from build123d import *

# Parameters (mm, degrees)
SKETCH1_R                         = 63.5
SKETCH1_R_2                       = 9.525
BOSS_EXTRUDE1_DEPTH               = 9.525
SKETCH4_R                         = 2.413
CUT_EXTRUDE1_DEPTH                = 10.525
CIRPATTERN1_COUNT                 = 8
SKETCH7_R                         = 33.02
BOSS_EXTRUDE4_DEPTH               = 4.826
SKETCH9_R                         = 33.02
CUT_EXTRUDE2_DEPTH                = 3.048
PIPE_TAP_DRILL_FOR_3_4_TAP4_D     = 23.0124
PIPE_TAP_DRILL_FOR_3_4_TAP4_DEPTH = 3.81
PIPE_TAP_DRILL_FOR_3_4_TAP4_TIP   = 6.913622455


with BuildPart() as part:
    # Sketch1 → Boss-Extrude1 (new body)
    with BuildSketch(Plane.XY):
        Circle(SKETCH1_R)
        Circle(SKETCH1_R_2, mode=Mode.SUBTRACT)
    extrude(amount=BOSS_EXTRUDE1_DEPTH)

    # Sketch4 → Cut-Extrude1 (cut, through all)
    with BuildSketch(Plane.XY.offset(9.525)):
        with Locations((49.866397767, 20.655338262)):
            Circle(SKETCH4_R)
    cut_extrude1 = extrude(amount=-CUT_EXTRUDE1_DEPTH, mode=Mode.SUBTRACT)

    # CirPattern1: Cut-Extrude1 ×8 about axis
    cirpattern1_axis = Axis((0, 0, 0), (0, 0, 1))
    for i in range(1, CIRPATTERN1_COUNT):
        add(cut_extrude1.rotate(cirpattern1_axis, i * 360 / CIRPATTERN1_COUNT), mode=Mode.SUBTRACT)

    # Sketch7 → Boss-Extrude4 (add)
    with BuildSketch(Plane.XY):
        with BuildLine():
            ThreePointArc((44.898742199, 0), (44.018213285, 2.330669915), (41.72653773, 3.308205888))
            Line((41.72653773, 3.308205888), (38.377645632, 3.308205888))
            ThreePointArc((38.377645632, 3.308205888), (36.132581602, 2.378269918), (35.202645632, 0.133205888))
            ThreePointArc((35.202645632, 0.133205888), (34.829644744, -0.48063442), (34.295865632, 0))
            add(Edge.make_bspline(
                [(34.295865632, 0), (34.29882834, 0.071916436), (34.304754577, 0.21576926), (34.311966888, 0.431642324), (34.317934755, 0.647612083), (34.327139988, 1.079917114), (34.332942166, 2.090306576), (34.279898225, 3.607362054), (34.120445155, 5.41030125), (33.960201682, 6.560746683), (33.865422793, 7.135076209), (33.865142183, 7.136775827)],
                knots=[0, 0, 0, 0, 0.000870248, 0.001740737, 0.002611466, 0.003482435, 0.006968712, 0.014826916, 0.02182843, 0.028845498, 0.028866325, 0.028866325, 0.028866325, 0.028866325], degree=3))
            add(Edge.make_bspline(
                [(33.865142183, 7.136775827), (33.7706713, 7.708973751), (33.552478291, 8.851599937), (33.138997804, 10.54970943), (32.639140351, 12.230302519), (32.054174895, 13.887355713), (31.385187056, 15.516557503), (30.633483645, 17.113645751), (29.800589951, 18.674419055), (28.8882464, 20.194747988), (27.898404875, 21.670586138), (26.833224521, 23.097980967), (25.695067067, 24.473084443), (24.486491635, 25.79216345), (23.210249051, 27.051609932), (21.869275652, 28.247950753), (20.466686605, 29.377857252), (19.005768742, 30.438154464), (17.489972932, 31.425829986), (15.922906004, 32.338042467), (14.30832223, 33.172129685), (12.650114403, 33.925616212), (10.95230451, 34.596220626), (9.219034045, 35.18186226), (7.454553956, 35.680667464), (5.663214286, 36.090975363), (3.849453494, 36.411343101), (2.017787512, 36.640550541), (0.172798549, 36.777604421), (-1.680876324, 36.82174194), (-3.538556782, 36.772433779), (-5.395531021, 36.629386524), (-7.247067665, 36.392544506), (-9.088427776, 36.062091031), (-10.914876942, 35.638449008), (-12.721697408, 35.122280961), (-14.504200214, 34.514488429), (-16.257737325, 33.816210747), (-17.977713699, 33.028823219), (-19.659599284, 32.153934663), (-21.298940898, 31.193384362), (-22.891373965, 30.149238397), (-24.43263408, 29.02378539), (-25.918568367, 27.819531655), (-27.345146601, 26.539195761), (-28.708472073, 25.185702541), (-30.004792148, 23.762176529), (-31.230508517, 22.271934869), (-32.382187085, 20.718479685), (-33.456567491, 19.105489956), (-34.450572223, 17.436812889), (-35.361315302, 15.716454831), (-36.186110516, 13.948571725), (-36.92247918, 12.137459144), (-37.568157395, 10.287541924), (-38.121102788, 8.403363415), (-38.579500717, 6.489574383), (-38.941769921, 4.550921586), (-39.206567586, 2.592236057), (-39.372793836, 0.618421113), (-39.439595611, -1.36555987), (-39.406369933, -3.354695889), (-39.272766542, -5.343940927), (-39.038689903, -7.328226707), (-38.704300556, -9.302475561), (-38.270015827, -11.261613379), (-37.736509879, -13.200582609), (-37.104713104, -15.11435526), (-36.375810853, -16.997945903), (-35.551241515, -18.846424601), (-34.632693929, -20.654929769), (-33.622104149, -22.418680905), (-32.521651558, -24.132991168), (-31.333754343, -25.793279776), (-30.061064337, -27.395084183), (-28.706461239, -28.934071999), (-27.273046228, -30.406052641), (-25.764134977, -31.806988658), (-24.18325009, -33.133006716), (-22.534112978, -34.380408214), (-20.820635184, -35.545679488), (-19.046909189, -36.625501594), (-17.217198713, -37.616759627), (-15.335928538, -38.516551562), (-13.407673866, -39.322196576), (-11.437149261, -40.031242854), (-9.429197172, -40.641474829), (-7.388776087, -41.15091985), (-5.32094834, -41.557854256), (-3.230867597, -41.86080884), (-1.123766056, -42.058573678), (0.995058608, -42.150202316), (3.120256518, -42.135015304), (5.246439066, -42.01260305), (7.368192535, -41.782828005), (9.480091844, -41.445826152), (11.576714375, -41.002007803), (13.652653862, -40.452057696), (15.702534288, -39.796934391), (17.72102376, -39.037868953), (19.702848338, -38.176362944), (21.642805765, -37.214185701), (23.535779073, -36.153370925), (25.376750026, -34.996212572), (27.16081237, -33.745260064), (28.883184839, -32.403312824), (30.539223912, -30.973414146), (32.12443625, -29.458844418), (33.634490817, -27.863113704), (35.065230621, -26.189953715), (36.412684063, -24.44330917), (37.673075861, -22.62732858), (38.842837509, -20.746354475), (39.91861725, -18.804913085), (40.897289536, -16.807703518), (41.775963949, -14.759586443), (42.55199355, -12.665572318), (43.22298264, -10.530809183), (43.786793912, -8.360570051), (44.241554967, -6.16023993), (44.571284542, -4.028278167), (44.740560267, -2.440845712), (44.813728039, -1.50376068), (44.839477521, -1.128293226), (44.857032226, -0.846470241), (44.872782179, -0.564469795), (44.886887576, -0.282309503), (44.894790326, -0.094111086), (44.898742199, 0)],
                knots=[0.028866325, 0.028866325, 0.028866325, 0.028866325, 0.035878186, 0.042926556, 0.049990663, 0.057070561, 0.064166299, 0.071277925, 0.078405484, 0.085549018, 0.092708569, 0.099884178, 0.107075882, 0.11428372, 0.121507729, 0.128747942, 0.136004396, 0.143277124, 0.150566158, 0.157871532, 0.165193276, 0.172531421, 0.179885999, 0.187257038, 0.194644569, 0.202048619, 0.209469218, 0.216906393, 0.224360171, 0.23183058, 0.239317647, 0.246821397, 0.254341857, 0.261879053, 0.269433009, 0.277003751, 0.284591303, 0.292195691, 0.299816937, 0.307455067, 0.315110103, 0.32278207, 0.33047099, 0.338176886, 0.345899781, 0.353639698, 0.361396658, 0.369170685, 0.376961799, 0.384770023, 0.392595378, 0.400437886, 0.408297568, 0.416174444, 0.424068536, 0.431979864, 0.439908449, 0.447854312, 0.455817472, 0.463797949, 0.471795764, 0.479810937, 0.487843486, 0.495893432, 0.503960795, 0.512045592, 0.520147845, 0.52826757, 0.536404789, 0.544559519, 0.552731779, 0.560921587, 0.569128963, 0.577353925, 0.58559649, 0.593856678, 0.602134505, 0.610429991, 0.618743153, 0.627074009, 0.635422576, 0.643788872, 0.652172916, 0.660574723, 0.668994312, 0.677431699, 0.685886903, 0.69435994, 0.702850826, 0.71135958, 0.719886217, 0.728430756, 0.736993211, 0.745573601, 0.754171941, 0.762788249, 0.771422539, 0.78007483, 0.788745137, 0.797433476, 0.806139864, 0.814864316, 0.823606849, 0.832367479, 0.841146221, 0.849943091, 0.858758106, 0.86759128, 0.87644263, 0.885312171, 0.894199918, 0.903105888, 0.912030094, 0.920972554, 0.929933282, 0.938912294, 0.947909603, 0.956925227, 0.96595918, 0.975011476, 0.984082132, 0.992034027, 0.994308583, 0.995446291, 0.996584287, 0.997722571, 0.998861142, 1, 1, 1, 1], degree=3))
        make_face()
        Circle(SKETCH7_R, mode=Mode.SUBTRACT)
        with BuildLine():
            ThreePointArc((35.202645632, 0.133205888), (36.132581602, 2.378269918), (38.377645632, 3.308205888))
            ThreePointArc((38.377645632, 3.308205888), (35.418733874, 4.394308044), (33.865142183, 7.136775827))
            add(Edge.make_bspline(
                [(34.295865632, 0), (34.29882834, 0.071916436), (34.304754577, 0.21576926), (34.311966888, 0.431642324), (34.317934755, 0.647612083), (34.327139988, 1.079917114), (34.332942166, 2.090306576), (34.279898225, 3.607362054), (34.120445155, 5.41030125), (33.960201682, 6.560746683), (33.865422793, 7.135076209), (33.865142183, 7.136775827)],
                knots=[0, 0, 0, 0, 0.000870248, 0.001740737, 0.002611466, 0.003482435, 0.006968712, 0.014826916, 0.02182843, 0.028845498, 0.028866325, 0.028866325, 0.028866325, 0.028866325], degree=3))
            ThreePointArc((34.295865632, 0), (34.829644744, -0.48063442), (35.202645632, 0.133205888))
        make_face()
    extrude(amount=-BOSS_EXTRUDE4_DEPTH)

    # Sketch9 → Cut-Extrude2 (cut)
    with BuildSketch(Plane(origin=(0, 0, 0), x_dir=(-1, 0, 0), z_dir=(0, 0, -1))):
        Circle(SKETCH9_R)
    extrude(amount=-CUT_EXTRUDE2_DEPTH, mode=Mode.SUBTRACT)

    # Pipe Tap Drill for 3/4 Tap4
    with Locations(Plane.XY.offset(9.525)):
        with Locations((0, 0)):
            Hole(PIPE_TAP_DRILL_FOR_3_4_TAP4_D / 2, depth=PIPE_TAP_DRILL_FOR_3_4_TAP4_DEPTH)
            with Locations((0, 0, -(PIPE_TAP_DRILL_FOR_3_4_TAP4_DEPTH + PIPE_TAP_DRILL_FOR_3_4_TAP4_TIP / 2))):  # 118° drill point
                Cone(0, PIPE_TAP_DRILL_FOR_3_4_TAP4_D / 2, PIPE_TAP_DRILL_FOR_3_4_TAP4_TIP, mode=Mode.SUBTRACT)


solid = part.part
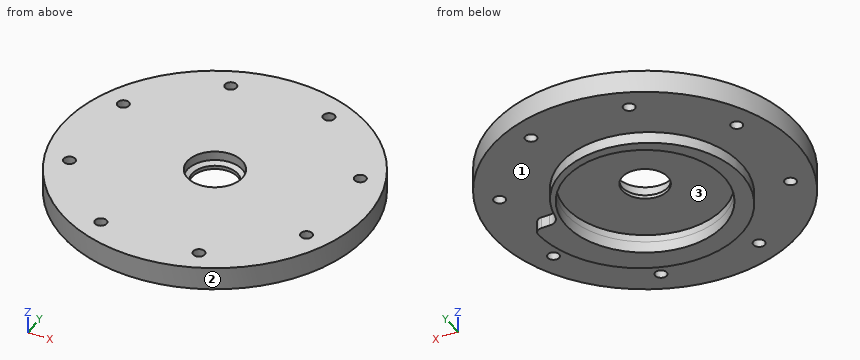
Verification items for the finished model (mm, model axes). Face numbers are marked on the shaded views. Coordinates: 2 decimals unless noted, no trailing zeros. Loops run counter-clockwise (first coordinate to the right, second up) from the corner with the lowest first, then second, coordinate; pieces in that order, holes last. Notation, with made-up numbers: (54.5, 86.5) -> (109.5, 86.5) arc R21 cw to (109.5, 116.5) -> close; hole circle Ø5 at (39, 67). An arc over 180 degrees is marked (long way). Write each question's results on one line, items separated by ' | '.
Item 1: Mould release check, pull along Y, two halves, no side actions. Record for the marked faces 1, 2 and 3: +Y half, -Y half, draft (parallel to the pull), parting line (faces both ways), or undercut.
Found:
face 1: draft | face 2: parting line | face 3: undercut
Item 2: Section check A-A, the plane x = -44.5. Enter the section's corners in (y, z) (3 decimals), plus the area to 3 significant figures.
Found:
outline: (-45.299, 0) -> (45.299, 0) -> (45.299, 9.525) -> (-45.299, 9.525) -> close | area: 863 mm2
Item 3: Material ranges on L1, parallel to Y at x = 0, z = 3.55 (3 decimals); L2, parallel to X at y = -20, z = 1.5; L3, parallel to X at y = 49.5, z = 5, recorded low to high.
Found:
L1: y = -63.5 to -9.525, 9.525 to 63.5 | L2: x = -60.27 to -52.19, -47.54 to -26.27, 26.27 to 47.54, 52.19 to 60.27 | L3: x = -39.77 to -23.04, -18.27 to 18.27, 23.04 to 39.77
Item 4: Gauge pin test, flat ends, axial feed: pin 1 (2 mm diameter, centred on y = -37.5, z = 7, fed in from +X); pin 2 (5.5 mm diameter, centred on x = -20.66, y = 49.87, fed in from -Z); pin 3 (3 mm diameter, centred on x = -49.87, y = -20.66, fed in from -Z); pin 4 (4 mm diameter, centred on x = 14.5, z = 3, fed in from -Y). Record the tip position at first contact, or that the pin passes through.
Found:
pin 1: stops at x = 51.96 | pin 2: stops at z = 0 | pin 3: passes through | pin 4: stops at y = -62.26
